Part model, mm, in its own coordinate system. Round coordinates to 2 decimals unless told otherwise and drop trailing zeros. Loops run counter-clockwise (first coordinate to the right, second up) from the corner with the lowest first, then second, coordinate; pieces in that order, holes last.
1) Band-saw the part on B-B, the plane z = -2.5. Write the cut outline in (x, y), then the cut area to 3 significant figures.
2) Band-saw the part on A-A, the plane x = -14. Write the cut outline in (y, z).
3) Band-saw the part on D-D, the plane x = 35. Write the cut outline in (y, z).
4) Mould opens along X. For faces 1 (the flat face through (-1, 0, -5)), 2 (the flat face through (-50, 0, -2)), 3 (the cylindrical face through (-33.522, 7.966, -2.465)) say: +X half, -X half, draft (parallel to the pull), parting line (faces both ways), or undercut.
5) Band-saw the part on C-C, the plane y = -12.5. Write the cut outline in (x, z), then the cut area to 3 significant figures.
6) Drop a flat-ended pin along its axis: P1, Ø10, axis at x = -11, y = -1.5, coming from the +Z side. Give the stop position or say it passes through.
7) Probe line 1 (Y direction, x = 35, z = -2.95); line 2 (Y direction, x = -14, z = -1.6). List the from-to ranges inside material, lowest first.
from build123d import *

# Parameters (mm, degrees)
ESQUISSE1_W        = 100
ESQUISSE1_H        = 45
ESQUISSE1_R        = 1.55
ESQUISSE1_R_2      = 4.05
BOSS_EXTRU_1_DEPTH = 5


with BuildPart() as part:
    # Esquisse1 → Boss.-Extru.1 (new body)
    with BuildSketch(Plane.XY):
        Rectangle(ESQUISSE1_W, ESQUISSE1_H)
        with Locations((-35, -12.5)):
            Circle(ESQUISSE1_R, mode=Mode.SUBTRACT)
        with Locations(Location((35, -12.5, 0), (0, 0, 180))):
            Circle(ESQUISSE1_R, mode=Mode.SUBTRACT)
        with Locations((14, 0)):
            Circle(ESQUISSE1_R_2, mode=Mode.SUBTRACT)
        with Locations(Location((-14, 0, 0), (0, 0, 180))):
            Circle(ESQUISSE1_R_2, mode=Mode.SUBTRACT)
        with Locations((-35, 7.5)):
            Circle(ESQUISSE1_R, mode=Mode.SUBTRACT)
        with Locations(Location((35, 7.5, 0), (0, 0, 180))):
            Circle(ESQUISSE1_R, mode=Mode.SUBTRACT)
    extrude(amount=-BOSS_EXTRU_1_DEPTH)


solid = part.part
Reported:
1. outline: (-50, -22.5) - (50, -22.5) - (50, 22.5) - (-50, 22.5) - close; hole circle Ø3.1 at (-35, -12.5); hole circle Ø3.1 at (-35, 7.5); hole circle Ø8.1 at (-14, 0); hole circle Ø8.1 at (14, 0); hole circle Ø3.1 at (35, -12.5); hole circle Ø3.1 at (35, 7.5)
1. area: 4,370 mm2
2. outline: (-22.5, -5) - (-4.05, -5) - (-4.05, 0) - (-22.5, 0) - close; (4.05, -5) - (22.5, -5) - (22.5, 0) - (4.05, 0) - close
3. outline: (-22.5, -5) - (-14.05, -5) - (-14.05, 0) - (-22.5, 0) - close; (-10.95, -5) - (5.95, -5) - (5.95, 0) - (-10.95, 0) - close; (9.05, -5) - (22.5, -5) - (22.5, 0) - (9.05, 0) - close
4. face 1: draft
4. face 2: -X half
4. face 3: undercut
5. outline: (-50, -5) - (-36.55, -5) - (-36.55, 0) - (-50, 0) - close; (-33.45, -5) - (33.45, -5) - (33.45, 0) - (-33.45, 0) - close; (36.55, -5) - (50, -5) - (50, 0) - (36.55, 0) - close
5. area: 469 mm2
6. P1: stops at z = 0
7. line 1: y = -22.5 to -14.05, -10.95 to 5.95, 9.05 to 22.5
7. line 2: y = -22.5 to -4.05, 4.05 to 22.5
